The listing builds one solid part. Answer for the finished solid, in the listing's coordinates (mm). Face numbers are marked on the shaded views. Round coordinates to 2 decimals unless told otherwise and drop trailing zeros. Write each loop counter-clockwise with the first axis right and the second up, starting at its lowest first coordinate (ties: lowest second). Pieces come first, ordered by that corner, then holes.
(1) A cutting plane is placed at B-B, the plane z = -7. Give the vertices of the cut face in (x, y) (3 decimals).
(2) Find the intervals of material crossed by probe 1 along X at (y, z) = (9.25, -2.25); probe 2 along X at (y, z) = (8.5, -10.25); probe 3 along X at (y, z) = (1, -17), in increasing order.
(3) A cutting plane is placed at C-C, the plane x = 106.53. Give the vertices of the cut face in (y, z), and give its area (3 significant figures).
(4) A cutting plane is placed at A-A, the plane y = 7.5. Give the vertices of the cut face in (x, z) (3 decimals), and give its area (3 significant figures).
(5) The mould has two halves that part along X. Classify the marked faces 1, 2, 3 and 4: +X half, -X half, draft (parallel to the pull), parting line (faces both ways), or undercut.
(6) A cutting plane is placed at D-D, the plane x = 119. Give the vertices of the cut face in (y, z), and give its area (3 significant figures).
from build123d import *

# Parameters (mm, degrees)
SKETCH_1_W          = 125
SKETCH_1_H          = 40
EXTRUDE_1_DEPTH     = 15
SKETCH_2_R          = 8.9
SKETCH_2_R_2        = 4.6
SKETCH_2_R_3        = 13.3
CUT_EXTRUDE_1_DEPTH = 133.098448136
CHAMFER_1_SIZE      = 1
CHAMFER_2_SIZE      = 1
FILLET_1_R          = 1
SKETCH_5_W          = 40
SKETCH_5_H          = 20
CUT_EXTRUDE_2_DEPTH = 133.098448148
FILLET_4_R          = 5
SKETCH_12_W         = 3.06
SKETCH_12_H         = 20
EXTRUDE_2_DEPTH     = 15
SKETCH_14_R         = 2.5
CUT_EXTRUDE_3_DEPTH = 128.47548784
SKETCH_15_W         = 36.94
SKETCH_15_H         = 20
EXTRUDE_3_DEPTH     = 15
SKETCH_16_W         = 106.425382254
SKETCH_16_H         = 56.336912026
CUT_EXTRUDE_4_DEPTH = 133.098448148
SKETCH_17_R         = 2.5
CUT_EXTRUDE_5_DEPTH = 133.098448136
SKETCH_18_R         = 4.6
CUT_EXTRUDE_6_DEPTH = 133.098448136
FILLET_5_R          = 1
SKETCH_19_W         = 47.376769249
SKETCH_19_H         = 22.00625663
CUT_EXTRUDE_7_DEPTH = 133.098448148
FILLET_6_R          = 1


with BuildPart() as part:
    # 草圖1 → 填料-伸長1 (new body)
    with BuildSketch(Plane(origin=(0, 0, 0), x_dir=(1, 0, 0), z_dir=(0, 1, 0))):
        with Locations((62.5, 20)):
            Rectangle(SKETCH_1_W, SKETCH_1_H)
    extrude(amount=EXTRUDE_1_DEPTH)

    # 草圖2 → 除料-伸長1 (cut, through all)
    with BuildSketch(Plane(origin=(0, 15, 0), x_dir=(1, 0, 0), z_dir=(0, 1, 0))):
        with Locations(Location((18.526668527, 20, 0), (0, 0, 270))):
            Circle(SKETCH_2_R)
        with Locations(Location((106.526668527, 20, 0), (0, 0, 270))):
            Circle(SKETCH_2_R_2)
        with Locations(Location((62.526668527, 20, 0), (0, 0, 270))):
            Circle(SKETCH_2_R_3)
    extrude(amount=-CUT_EXTRUDE_1_DEPTH, mode=Mode.SUBTRACT)

    # 導角1
    chamfer_1_edges = [part.edges().sort_by_distance(p)[0] for p in [
        (18.526668527, 15, -28.9),
    ]]
    chamfer(chamfer_1_edges, length=CHAMFER_1_SIZE)

    # 導角2
    chamfer_2_edges = [part.edges().sort_by_distance(p)[0] for p in [
        (18.526668527, 0, -28.9),
    ]]
    chamfer(chamfer_2_edges, length=CHAMFER_2_SIZE)

    # 圓角1
    fillet_1_edges = [part.edges().sort_by_distance(p)[0] for p in [
        (106.526668527, 0, -24.6),
        (106.526668527, 15, -24.6),
        (62.526668527, 0, -33.3),
        (62.526668527, 15, -33.3),
    ]]
    fillet(fillet_1_edges, radius=FILLET_1_R)

    # 草圖5 → 除料-伸長2 (cut, through all)
    with BuildSketch(Plane(origin=(0, 15, 0), x_dir=(1, 0, 0), z_dir=(0, 1, 0))):
        with Locations((105, 10)):
            Rectangle(SKETCH_5_W, SKETCH_5_H)
    extrude(amount=-CUT_EXTRUDE_2_DEPTH, mode=Mode.SUBTRACT)

    # 圓角4
    fillet_4_edges = [part.edges().sort_by_distance(p)[0] for p in [
        (0, 7.5, -40),
        (0, 7.5, 0),
    ]]
    fillet(fillet_4_edges, radius=FILLET_4_R)

    # 草圖12 → 填料-伸長2 (add)
    with BuildSketch(Plane(origin=(0, 15, 0), x_dir=(1, 0, 0), z_dir=(0, 1, 0))):
        with Locations((86.53, 10)):
            Rectangle(SKETCH_12_W, SKETCH_12_H)
    extrude(amount=-EXTRUDE_2_DEPTH)

    # 草圖14 → 除料-伸長3 (cut, through all)
    with BuildSketch(Plane.XY.offset(-20)):
        with Locations((118.565, 7.5)):
            Circle(SKETCH_14_R)
        with Locations((95.491668527, 7.5)):
            Circle(SKETCH_14_R)
    extrude(amount=-CUT_EXTRUDE_3_DEPTH, mode=Mode.SUBTRACT)

    # 草圖16 → 除料-伸長4 (cut, through all)
    with BuildSketch(Plane(origin=(0, 15, 0), x_dir=(1, 0, 0), z_dir=(0, 1, 0))):
        with Locations((34.847308873, 28.168456013)):
            Rectangle(SKETCH_16_W, SKETCH_16_H)
    extrude(amount=-CUT_EXTRUDE_4_DEPTH, mode=Mode.SUBTRACT)


with BuildPart() as body_2:
    # 草圖15 → 填料-伸長3 (new body)
    with BuildSketch(Plane(origin=(0, 15, 0), x_dir=(1, 0, 0), z_dir=(0, 1, 0))):
        with Locations((106.53, 10)):
            Rectangle(SKETCH_15_W, SKETCH_15_H)
    extrude(amount=-EXTRUDE_3_DEPTH)

    # 草圖17 → 除料-伸長5 (cut, through all)
    with BuildSketch(Plane.XY):
        with Locations((95.491668527, 7.5)):
            Circle(SKETCH_17_R)
        with Locations((118.565, 7.5)):
            Circle(SKETCH_17_R)
    extrude(amount=-CUT_EXTRUDE_5_DEPTH, mode=Mode.SUBTRACT)


with BuildPart() as cut_extrude_6_tool:
    # 草圖18 → 除料-伸長6 (new, through all)
    with BuildSketch(Plane(origin=(0, 15, 0), x_dir=(1, 0, 0), z_dir=(0, 1, 0))):
        with Locations((106.53, 20)):
            Circle(SKETCH_18_R)
    extrude(amount=-CUT_EXTRUDE_6_DEPTH)


with BuildPart() as part_1:
    add(part.part)

    # 除料-伸長6: cut by cut_extrude_6_tool
    add(cut_extrude_6_tool.part, mode=Mode.SUBTRACT)

    # 草圖19 → 除料-伸長7 (cut, through all)
    with BuildSketch(Plane(origin=(0, 15, 0), x_dir=(1, 0, 0), z_dir=(0, 1, 0))):
        with Locations((111.748384625, 31.003128315)):
            Rectangle(SKETCH_19_W, SKETCH_19_H)
    extrude(amount=-CUT_EXTRUDE_7_DEPTH, mode=Mode.SUBTRACT)


with BuildPart() as body_2_1:
    add(body_2.part)

    # 除料-伸長6: cut by cut_extrude_6_tool
    add(cut_extrude_6_tool.part, mode=Mode.SUBTRACT)

    # 圓角5
    fillet_5_edges = [body_2_1.edges().sort_by_distance(p)[0] for p in [
        (106.53, 15, -15.4),
    ]]
    fillet(fillet_5_edges, radius=FILLET_5_R)

    # 圓角6
    fillet_6_edges = [body_2_1.edges().sort_by_distance(p)[0] for p in [
        (106.53, 0, -15.4),
    ]]
    fillet(fillet_6_edges, radius=FILLET_6_R)


solid = body_2_1.part
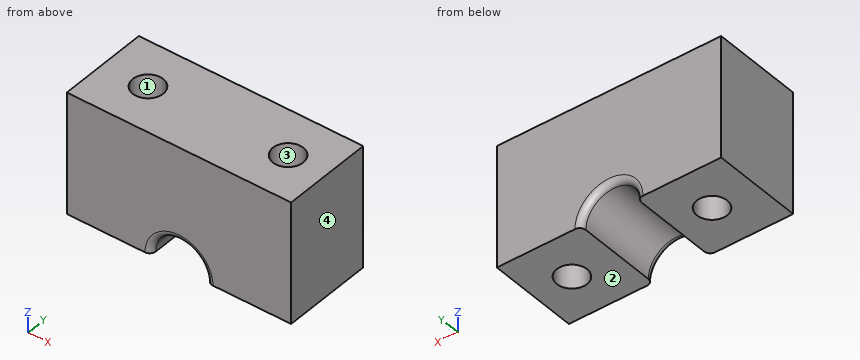
Solutions:
1. outline: (88.06, 0) - (125, 0) - (125, 15) - (88.06, 15) - close; hole circle Ø5 at (95.492, 7.5); hole circle Ø5 at (118.565, 7.5)
2. probe 1: x = 88.06 to 93.71, 97.28 to 116.78, 120.35 to 125
2. probe 2: x = 88.06 to 93.2, 97.78 to 116.27, 120.86 to 125
2. probe 3: x = 88.06 to 103.04, 110.02 to 125
3. outline: (0, -14.4) arc R1 ccw to (1, -15.4) - (14, -15.4) arc R1 ccw to (15, -14.4) - (15, 0) - (0, 0) - close
3. area: 231 mm2
4. outline: (88.06, -20) - (92.992, -20) - (92.992, 0) - (88.06, 0) - close; (97.992, -20) - (101.93, -20) arc R4.6 cw to (111.13, -20) - (116.065, -20) - (116.065, 0) - (97.992, 0) - close; (121.065, -20) - (125, -20) - (125, 0) - (121.065, 0) - close
4. area: 506 mm2
5. face 1: undercut
5. face 2: draft
5. face 3: undercut
5. face 4: +X half
6. outline: (0, -20) - (5.04, -20) - (5.04, 0) - (0, 0) - close; (9.96, -20) - (15, -20) - (15, 0) - (9.96, 0) - close
6. area: 202 mm2
